Autodesk Inventor part; units mm, degrees
ref_plane "YZ Plane" through (0, 0, 0) normal (1, 0, 0) x (0, 1, 0)
ref_plane "XZ Plane" through (0, 0, 0) normal (0, 1, 0) x (-1, 0, 0)
ref_plane "XY Plane" through (0, 0, 0) normal (0, 0, 1) x (1, 0, 0)
sketch "Base" plane through (0, 0, 0) normal (0, 1, 0) x (-1, 0, 0)
  line L0 (0, 25) -> (0, -175)
  line L1 (0, -175) -> (54, -175)
  line L2 (54, -175) -> (54, 25)
  line L3 (54, 25) -> (0, 25)
  dimension "d6" = 200
  dimension "d7" = 54
extrude "Extrusion2" add sketch "Base" along normal blind 45
sketch "Top" plane through (0, 45, 0) normal (0, 1, 0) x (1, 0, 0)
  circle A0 centre (-27, 51) radius 14.25
  circle A1 centre (-27, 3) radius 14.25
  circle A2 centre (-27, 99) radius 14.25
  circle A3 centre (-27, 147) radius 14.25
  line L0 (0, 175) -> (-54, 175)
  line L1 (-54, 175) -> (-54, -25)
  line L2 (-54, -25) -> (0, -25) construction
  line L3 (-27, -25) -> (-27, 175) construction
  circle A4 centre (-27, 3) radius 11.4
  circle A5 centre (-27, 51) radius 11.4
  circle A6 centre (-27, 99) radius 11.4
  circle A7 centre (-27, 147) radius 11.4
  point P0 (-27, 75)
  dimension "d10" = 28.5
  dimension "d11" = 28.5
  dimension "d12" = 28.5
  dimension "d13" = 28.5
  dimension "d14" = 48
  dimension "d15" = 48
  dimension "d16" = 48
  dimension "d27" = 22.8
  dimension "d28" = 22.8
  dimension "d29" = 22.8
  dimension "d30" = 22.8
  dimension "d31" = 24
  dimension "d32" = 100
  dimension "d35" = 28
extrude "Extrusion3" cut sketch "Top" against normal up to next contours A4 | A5 | A6 | A7
sketch "Walls" plane through (0, 0, 0) normal (0, -1, 0) x (1, 0, 0)
  line L0 (-8, 17) -> (-46, 17)
  line L1 (-46, 17) -> (-46, -167)
  line L2 (-46, -167) -> (-8, -167)
  line L3 (-8, -167) -> (-8, 17)
  line L4 (-54, 25) -> (0, 25)
  line L5 (0, -175) -> (-54, -175)
  line L6 (0, 25) -> (0, -175)
  line L7 (-54, -175) -> (-54, 25)
  point P0 (0, 0)
  dimension "d21" = 8
  dimension "d22" = 8
  dimension "d23" = 8
  dimension "d24" = 8
  dimension "d33" = 38
extrude "Extrusion4" cut sketch "Walls" against normal blind 33 contours L3 L2 L1 L0
fillet "Fillet1" radius 12 8 edges at (-27, 45, 25) (-54, 45, -75) (0, 45, -75) (0, 22.5, 25) (-54, 22.5, 25) (0, 22.5, -175) (-27, 45, -175) (-54, 22.5, -175)
sketch "Sketch7" plane through (-54, 0, -163) normal (-1, 0, 0) x (0, 0, 1)
  line L0 (0, 33) -> (176, 33)
  line L1 (0, 0) -> (176, 0)
  circle A0 centre (88, 0) radius 3
  point P0 (163, 0)
  dimension "d40" = 6
extrude "Extrusion5" cut sketch "Sketch7" against normal up to surface (8 mm away)
fillet "Fillet2" radius 5 4 edges at (-8, 16.5, 17) (-46, 16.5, 17) (-8, 16.5, -167) (-46, 16.5, -167)
sketch "Sketch10" plane through (-12, 0, -175) normal (0, 0, -1) x (-1, 0, 0)
  line L0 (83.179, 90.3723) -> (-24.5359, 90.3723)
  line L1 (-24.5359, 90.3723) -> (-24.5359, -32.2986)
  line L2 (-24.5359, -32.2986) -> (83.179, -32.2986)
  line L3 (83.179, -32.2986) -> (83.179, 90.3723)
  point P0 (-12, 0)
extrude "Half" cut sketch "Sketch10" against normal blind 100
sketch "Sketch13" plane through (0, 0, 0) normal (0, -1, 0) x (1, 0, 0)
  line L0 (-8, 12) -> (-8, -75)
  line L1 (-8, -51) -> (-4, -51)
  line L2 (-4, -51) -> (-4, -43)
  line L3 (-4, -43) -> (-8, -43)
  line L4 (-8, -43) -> (-8, -51)
  circle A0 centre (-27, -51) radius 11.4 construction
  line L5 (0, 13) -> (0, -75) construction
  line L6 (0, -35) -> (-53.8786, -35) construction
  circle A1 centre (-27, -3) radius 11.4 construction
  line L7 (-8, -82) -> (-8, 5)
  line L8 (-8, -19) -> (-4, -19)
  line L9 (-4, -19) -> (-4, -27)
  line L10 (-4, -27) -> (-8, -27)
  line L11 (-8, -27) -> (-8, -19)
  line L12 (-27, -51) -> (-27, -3) construction
  line L13 (-46, -51) -> (-50, -51)
  line L14 (-50, -51) -> (-50, -43)
  line L15 (-50, -43) -> (-46, -43)
  line L16 (-46, -43) -> (-46, -51)
  line L17 (-46, -19) -> (-50, -19)
  line L18 (-46, -27) -> (-46, -19)
  line L19 (-50, -19) -> (-50, -27)
  line L20 (-50, -27) -> (-46, -27)
  point P0 (0, 0)
  point P1 (-8, -19)
  point P2 (-8, -27)
  point P3 (-8, -43)
  dimension "d50" = 4
  dimension "d52" = 8
  dimension "d53" = 0
  dimension "d54" = 8
extrude "Extrusion7" cut sketch "Sketch13" against normal blind 5
equation "\"d11\" = d10"
equation "\"d12\" = d10"
equation "\"d13\" = d10"
equation "\"d15\" = d14"
equation "\"d16\" = d14"
equation "\"d28\" = d27"
equation "\"d29\" = d27"
equation "\"d30\" = d27"
equation "\"d22\" = d21"
equation "\"d23\" = d21"
equation "\"d24\" = d23"
properties part number "_3DPrint"
Could you check a few things on this model? Use its own coordinates, in mm. A direction names the side the tool comes from. Give positions to 0.01 mm unless a question says otherwise; leave off trailing zeros. Write each loop counter-clockwise with the first axis right and the second up, starting at its lowest first coordinate (ties: lowest second). Pieces come first, ordered by that corner, then holes. Notation, with made-up numbers: (-4, 81) -> (48, 81) arc R7 cw to (48, 92) -> close; hole circle Ø1 at (-17.75, -9.75). An arc over 180 degrees is marked (long way). Answer as CSV lines item,"result". Start each with the question number.
(1) Which directions (+Z, -Z, +X, -X, +Y, -Y) give clear straight access to the entire face, cutting with the end or side of a thin tool? Please do faces 1 (the face through (-50.39, 41.58, -30.38)), 2 (the face through (-48, 2, -51)), 3 (the face through (-10, 17, 16)).
(2) If we section it at B-B, the plane x = -27: Write out the boundary of the cut face in (y, z), and give its area (3 significant figures).
(3) I'm going to push flat-ended pins straight in: pin 1 Ø4.5 at (x, z) = (-6.5, -47) entering from -Y; pin 2 Ø3 at (x, y) = (-48.5, 1.5) entering from +Z; pin 3 Ø11.5 at (x, z) = (-36.5, -18.5) entering from -Y; pin 4 Ø20.5 at (x, z) = (-27, -3) entering from -Y. Where does each tip first touch, or does it pass through?
(4) Please list where these lines run through material, in increasing order: line 1 (Z direction, x = -27, y = 41.25); line 2 (Z direction, x = -27, y = 38.5); line 3 (X direction, y = 25.5, z = -60.5).
(5) If we section it at C-C, the plane y = 35: Write out the boundary of the cut face in (x, z).
(6) If we section it at D-D, the plane z = 10: Write out the boundary of the cut face in (x, y).
(7) If we mould it in two halves opening along X, with no side actions, what happens to faces 4 (the face through (-26.79, 41.58, 21.39)), 5 (the face through (-4, 2, -47)), 6 (the face through (-3.61, 41.58, -31.62)), 7 (the face through (-27, 33, -28))? For each: +X half, -X half, draft (parallel to the pull), parting line (faces both ways), or undercut.
(8) If we section it at A-A, the plane z = -3: Write out the boundary of the cut face in (x, y).
Answer list:
1,face 1,"+Z, -Z, -X, +Y"
1,face 2,"-Y"
1,face 3,"-Z, -Y"
2,outline,"(0, 17) -> (33, 17) -> (33, 8.4) -> (45, 8.4) -> (45, 13) arc R12 ccw to (33, 25) -> (0, 25) -> close; (33, -75) -> (45, -75) -> (45, -62.4) -> (33, -62.4) -> close; (33, -39.6) -> (45, -39.6) -> (45, -14.4) -> (33, -14.4) -> close"
2,area,"886 mm^2"
3,pin 1,"y = 5"
3,pin 2,"z = 23.91"
3,pin 3,"y = 33"
3,pin 4,"through"
4,line 1,"-75 to -62.4, -39.6 to -14.4, 8.4 to 21.71"
4,line 2,"-75 to -62.4, -39.6 to -14.4, 8.4 to 23.67"
4,line 3,"-54 to -46, -8 to 0"
5,outline,"(-53.83, -75) -> (-0.17, -75) -> (-0.17, 13) arc R11.83 ccw to (-12, 24.83) -> (-42, 24.83) arc R11.83 ccw to (-53.83, 13) -> close; hole circle Ø22.8 at (-27, -51); hole circle Ø22.8 at (-27, -3)"
6,outline,"(-54, 0) -> (-46, 0) -> (-46, 33) -> (-8, 33) -> (-8, 0) -> (0, 0) -> (0, 33) arc R12 ccw to (-12, 45) -> (-42, 45) arc R12 ccw to (-54, 33) -> close"
7,face 4,"draft"
7,face 5,"undercut"
7,face 6,"+X half"
7,face 7,"undercut"
8,outline,"(-54, 0) -> (-46, 0) -> (-46, 33) -> (-38.4, 33) -> (-38.4, 45) -> (-42, 45) arc R12 ccw to (-54, 33) -> close; (-15.6, 33) -> (-8, 33) -> (-8, 0) -> (0, 0) -> (0, 33) arc R12 ccw to (-12, 45) -> (-15.6, 45) -> close"
